Geometry: final body of the model. Coordinates: model frame, mm. Coordinates: 2 decimals unless noted, no trailing zeros. Write each loop counter-clockwise with the first axis right and the second up, starting at its lowest first coordinate (ties: lowest second). Pieces come first, ordered by that corner, then holes. Notation, with made-up numbers: (42.25, 34) -> (52.25, 34) arc R22 cw to (52.25, 58) -> close; hole circle Ø4 at (-38, -18). An arc over 180 degrees is marked (long way). One line per item, written item: value. Start each with the question number.
from build123d import *

# Parameters (mm, degrees)
SKETCH1_W           = 80
SKETCH1_H           = 80
BOSS_EXTRUDE1_DEPTH = 1.5875
SKETCH2_OUTSIDE_W   = 104.636
SKETCH2_OUTSIDE_H   = 104.636
CUT_EXTRUDE2_DEPTH  = 10
SKETCH3_W           = 80
SKETCH3_H           = 48.498076923
CUT_EXTRUDE3_DEPTH  = 57.657573413


with BuildPart() as part:
    # Sketch1 → Boss-Extrude1 (new, symmetric)
    with BuildSketch(Plane.XY):
        Rectangle(SKETCH1_W, SKETCH1_H)
    extrude(amount=BOSS_EXTRUDE1_DEPTH, both=True)

    # Sketch2 outside → Cut-Extrude2 (cut)
    with BuildSketch(Plane.XY.offset(1.5875)):
        Rectangle(SKETCH2_OUTSIDE_W, SKETCH2_OUTSIDE_H)
        Polygon((33.846153846, -36.825), (40, -36.825), (40, -31.159615385), (36.82, -31.159615385), (36.82, -25.494230769), (40, -25.494230769), (40, -19.828846154), (36.82, -19.828846154), (36.82, -14.163461538), (40, -14.163461538), (40, -8.498076923), (36.82, -8.498076923), (36.82, -2.832692308), (40, -2.832692308), (40, 2.832692308), (36.82, 2.832692308), (36.82, 8.498076923), (40, 8.498076923), (40, 14.163461538), (36.82, 14.163461538), (36.82, 19.828846154), (40, 19.828846154), (40, 25.494230769), (36.82, 25.494230769), (36.82, 31.159615385), (40, 31.159615385), (40, 36.825), (33.846153846, 36.825), (33.846153846, 40), (27.692307692, 40), (27.692307692, 36.825), (21.538461538, 36.825), (21.538461538, 40), (15.384615385, 40), (15.384615385, 36.825), (9.230769231, 36.825), (9.230769231, 40), (3.076923077, 40), (3.076923077, 36.825), (-3.076923077, 36.825), (-3.076923077, 40), (-9.230769231, 40), (-9.230769231, 36.825), (-15.384615385, 36.825), (-15.384615385, 40), (-21.538461538, 40), (-21.538461538, 36.825), (-27.692307692, 36.825), (-27.692307692, 40), (-33.846153846, 40), (-33.846153846, 36.825), (-40, 36.825), (-40, 31.159615385), (-36.82, 31.159615385), (-36.82, 25.494230769), (-40, 25.494230769), (-40, 19.828846154), (-36.82, 19.828846154), (-36.82, 14.163461538), (-40, 14.163461538), (-40, 8.498076923), (-36.82, 8.498076923), (-36.82, 2.832692308), (-40, 2.832692308), (-40, -2.832692308), (-36.82, -2.832692308), (-36.82, -8.498076923), (-40, -8.498076923), (-40, -14.163461538), (-36.82, -14.163461538), (-36.82, -19.828846154), (-40, -19.828846154), (-40, -25.494230769), (-36.82, -25.494230769), (-36.82, -31.159615385), (-40, -31.159615385), (-40, -36.825), (-33.846153846, -36.825), (-33.846153846, -40), (-27.692307692, -40), (-27.692307692, -36.825), (-21.538461538, -36.825), (-21.538461538, -40), (-15.384615385, -40), (-15.384615385, -36.825), (-9.230769231, -36.825), (-9.230769231, -40), (-3.076923077, -40), (-3.076923077, -36.825), (3.076923077, -36.825), (3.076923077, -40), (9.230769231, -40), (9.230769231, -36.825), (15.384615385, -36.825), (15.384615385, -40), (21.538461538, -40), (21.538461538, -36.825), (27.692307692, -36.825), (27.692307692, -40), (33.846153846, -40), align=None, mode=Mode.SUBTRACT)
    extrude(amount=-CUT_EXTRUDE2_DEPTH, mode=Mode.SUBTRACT)

    # Sketch3 → Cut-Extrude3 (cut, through all)
    with BuildSketch(Plane.XY.offset(1.5875)):
        with Locations((0, -15.750961539)):
            Rectangle(SKETCH3_W, SKETCH3_H)
    extrude(amount=-CUT_EXTRUDE3_DEPTH, mode=Mode.SUBTRACT)


solid = part.part
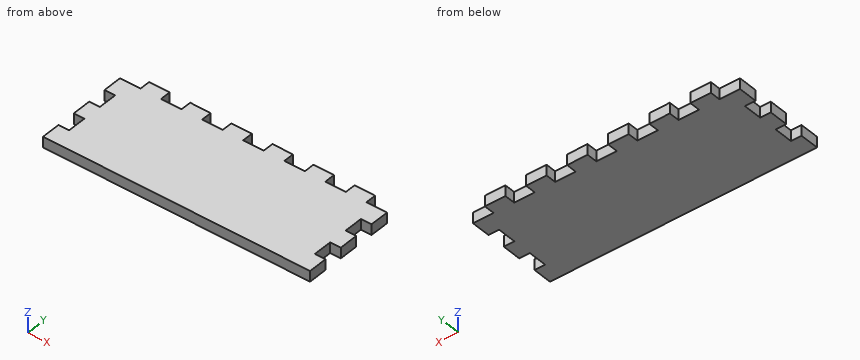
Q1. First-contact query: P1, Ø1.6, axis at y = 38, z = 0, coming from the +X side; P2, Ø1.6, axis at y = 29, z = 0.5, coming from the -X side; P3, Ø1.6, axis at y = 38.5, z = -0.5, coming from the -X side. Flat tips, straight axial feed; report the tip coordinate or a pass-through.
Q2. Cut plane B-B on y = 27. Output: boundary loops of the cut face in (x, z), and give its area (3 significant figures).
Q3. Line query: L1, parallel to X at y = 37.5, z = -0.9; L2, parallel to Y at x = -2.5, z = -0.5 (3 decimals); L3, parallel to X at y = 30, z = 1.45. Output: solid intervals per line, ascending. Write a range as from..to.
Q4. Cut plane A-A on x = 35.5. Output: boundary loops of the cut face in (y, z) (1 decimal), and give its area (3 significant figures).
Solution:
1. P1: x = 33.85
1. P2: x = -36.82
1. P3: x = -33.85
2. outline: (-36.82, -1.59) -> (36.82, -1.59) -> (36.82, 1.59) -> (-36.82, 1.59) -> close
2. area: 234 mm²
3. L1: -33.85..-27.69, -21.54..-15.38, -9.23..-3.08, 3.08..9.23, 15.38..21.54, 27.69..33.85
3. L2: 8.498..36.825
3. L3: -36.82..36.82
4. outline: (8.5, -1.6) -> (36.8, -1.6) -> (36.8, 1.6) -> (8.5, 1.6) -> close
4. area: 89.9 mm²
